The model under review builds one solid part; all positions refer to its coordinate system, in mm. A direction names the side the tool comes from. Coordinates: 2 decimals unless noted, no trailing zeros. Order: outer loops, then holes, each group sorted by start corner. A loop starts at its lowest first (then second) coordinate and runs counter-clockwise, first axis right, second up. Notation, with made-up numbers: M -7,-3 L 20,-3 A17 ccw 20,15 Z; hole C 50,79 d5. An arc over 180 degrees is marked long. One line per item, written item: value.
```python
from build123d import *

# Parameters (mm, degrees)
F0_W     = 101.6
F0_H     = 50.8
F1_DEPTH = 25.4
F2_R     = 6.35
F2_R_2   = 6.933717
F3_DEPTH = 25.401
F4_W     = 40.821289
F4_H     = 26.813686


with BuildPart() as f1:
    # F0 (on Right) → F1 (new body)
    with BuildSketch(Plane.YZ):
        Rectangle(F0_W, F0_H)
    extrude(amount=F1_DEPTH)

    # F2 (on face) → F3 (cut, through all)
    with BuildSketch(Plane.YZ.offset(25.4)):
        with Locations((-38.1, 15.86114)):
            Circle(F2_R)
        with Locations((38.1, 15.86114)):
            Circle(F2_R)
        with Locations((38.1, -9.666498)):
            Circle(F2_R_2)
        with Locations((-38.1, -9.666498)):
            Circle(F2_R_2)
    extrude(amount=-F3_DEPTH, mode=Mode.SUBTRACT)

    # F4 (on Top) → F5 (revolve)
    with BuildSketch(Plane.XY):
        with Locations((45.810644, -13.406843)):
            Rectangle(F4_W, F4_H)
    revolve(axis=Axis((45.810645, 0, 0), (-1, 0, 0)))


solid = f1.part
```
(1) Mouldability with a two-part tool opening along Z and no side actions: class faces 3 (the flat face through (25.4, 34, 0)), 4 (the flat face through (13, -1, -25.4)), 5 (the cylindrical face through (12.878, 31.756, 16.14)) as +Z half, -Z half, draft (parallel to the pull), parting line (faces both ways), or undercut.
Geometry results:
face 3: draft
face 4: -Z half
face 5: undercut
(2) For L1, parallel to Z at x = 11.75, y = 38.1; L2, parallel to Y at x = 3, z = 15; L3, parallel to Y at x = 22, z = 20, list the stretches that pass through material, from the lowest coordinate up.
Geometry results:
L1: z = -25.4 to -16.6, -2.73 to 9.51, 22.21 to 25.4
L2: y = -50.8 to -44.39, -31.81 to 31.81, 44.39 to 50.8
L3: y = -50.8 to -42.92, -33.28 to 33.28, 42.92 to 50.8
(3) We need section B-B, the plane z = 18. State the section outline as (x, y) points, plus the area to 3 significant figures.
Geometry results:
outline: M 0,-50.8 L 25.4,-50.8 L 25.4,-44.08 L 0,-44.08 Z; M 0,-32.12 L 25.4,-32.12 L 25.4,-19.87 L 66.22,-19.87 L 66.22,19.87 L 25.4,19.87 L 25.4,32.12 L 0,32.12 Z; M 0,44.08 L 25.4,44.08 L 25.4,50.8 L 0,50.8 Z
area: 3,600 mm2
(4) Tool access review of faces 1 (the cylindrical face through (46.096, 26.788, 1.179)), 2 (the flat face through (66.221, 0, 0)): name each direction out of +Z, -Z, +X, -X, +Y, -Y from which nothing blocks a thin tool from reaching the whole face with its end or side.
Geometry results:
face 1: +X
face 2: +Z, -Z, +X, +Y, -Y
(5) We need section D-D, the plane x = 6. State the section outline as (y, z) points, plus the area to 3 significant figures.
Geometry results:
outline: M -50.8,-25.4 L 50.8,-25.4 L 50.8,25.4 L -50.8,25.4 Z; hole C -38.1,-9.67 d13.87; hole C -38.1,15.86 d12.7; hole C 38.1,-9.67 d13.87; hole C 38.1,15.86 d12.7
area: 4,610 mm2
(6) Insertion check: pin 1 Ø4 at (x, z) = (31.5, 4) entering from -Y; pin 2 Ø7.5 at (x, y) = (16.5, 22.5) entering from -Z; pin 3 Ø3 at (x, z) = (33, -15.5) entering from +Y. Each pin has a flat end and moves straight along its axis. Give the tip position at first contact, or say it passes through.
Geometry results:
pin 1: stops at y = -26.74
pin 2: stops at z = -25.4
pin 3: stops at y = 22.87
(7) We need section A-A, the plane y = -38.1. State the section outline as (x, z) points, plus the area to 3 significant figures.
Geometry results:
outline: M 0,-25.4 L 25.4,-25.4 L 25.4,-16.6 L 0,-16.6 Z; M 0,-2.73 L 25.4,-2.73 L 25.4,9.51 L 0,9.51 Z; M 0,22.21 L 25.4,22.21 L 25.4,25.4 L 0,25.4 Z
area: 616 mm2
(8) We need section C-C, the plane y = 0. State the section outline as (x, z) points, plus the area to 3 significant figures.
Geometry results:
outline: M 0,-25.4 L 25.4,-25.4 L 25.4,-26.81 L 66.22,-26.81 L 66.22,26.81 L 25.4,26.81 L 25.4,25.4 L 0,25.4 Z
area: 3,480 mm2
